```python
from build123d import *

# Parameters (mm, degrees)
F1_DEPTH  = 3.175
F2_R      = 3.556
F3_DEPTH  = 25.4
F4_DEPTH  = 25.4
F2_R_2    = 6.35
F5_DEPTH  = 25.4
F6_DEPTH  = 25.4
F7_DEPTH  = 25.4
F8_DEPTH  = 25.4
F9_R      = 18.9992
F9_R_2    = 1.8542
F10_DEPTH = 25.4


with BuildPart() as f1:
    # F0 (on Top) → F1 (new body)
    with BuildSketch(Plane.XY):
        Polygon((0, 31.75), (0, 101.6), (-444.5, 101.6), (-444.5, 31.75), (-412.75, 0), (-31.75, 0), align=None)
    extrude(amount=F1_DEPTH)

    # F2 (on face) → F3 (cut)
    with BuildSketch(Plane.XY.offset(3.175)):
        with Locations((-438.15, 50.8)):
            Circle(F2_R)
    extrude(amount=-F3_DEPTH, mode=Mode.SUBTRACT)

    # F2 (on face) → F4 (cut)
    with BuildSketch(Plane.XY.offset(3.175)):
        with Locations((-438.15, 76.2)):
            Circle(F2_R)
    extrude(amount=-F4_DEPTH, mode=Mode.SUBTRACT)

    # F2 (on face) → F5 (cut)
    with BuildSketch(Plane.XY.offset(3.175)):
        with Locations((-381, 31.75)):
            Circle(F2_R_2)
    extrude(amount=-F5_DEPTH, mode=Mode.SUBTRACT)

    # F2 (on face) → F6 (cut)
    with BuildSketch(Plane.XY.offset(3.175)):
        with Locations((-63.5, 31.75)):
            Circle(F2_R_2)
    extrude(amount=-F6_DEPTH, mode=Mode.SUBTRACT)

    # F2 (on face) → F7 (cut)
    with BuildSketch(Plane.XY.offset(3.175)):
        with Locations((-6.35, 76.2)):
            Circle(F2_R)
    extrude(amount=-F7_DEPTH, mode=Mode.SUBTRACT)

    # F2 (on face) → F8 (cut)
    with BuildSketch(Plane.XY.offset(3.175)):
        with Locations((-6.35, 50.8)):
            Circle(F2_R)
    extrude(amount=-F8_DEPTH, mode=Mode.SUBTRACT)

    # F9 (on face) → F10 (cut)
    with BuildSketch(Plane.XY.offset(3.175)):
        with Locations((-314.325, 31.75)):
            Circle(F9_R)
        with Locations((-338.328, 38.7604)):
            Circle(F9_R_2)
        with Locations((-290.322, 38.7604)):
            Circle(F9_R_2)
        with Locations((-130.175, 31.75)):
            Circle(F9_R)
        with Locations((-154.178, 38.7604)):
            Circle(F9_R_2)
        with Locations((-106.172, 38.7604)):
            Circle(F9_R_2)
    extrude(amount=-F10_DEPTH, mode=Mode.SUBTRACT)


solid = f1.part
```
Could you check a few things on this model? Use its own coordinates, in mm. Give positions to 0.01 mm unless a question says otherwise; leave off trailing zeros. Loops run counter-clockwise (first coordinate to the right, second up) from the corner with the lowest first, then second, coordinate; pieces in that order, holes last. Notation, with made-up numbers: (19.5, -16) -> (33.5, -16) arc R18 cw to (33.5, 15) -> close; hole circle Ø3 at (-31, 86.25). An arc over 180 degrees is marked (long way). Put each result on its own line as item: value.
(1) Imagine slicing it at A-A on x = -63.5. Write out the boundary of the cut face in (y, z) (3 decimals), plus the area to 3 significant figures.
Computed:
outline: (0, 0) -> (25.4, 0) -> (25.4, 3.175) -> (0, 3.175) -> close; (38.1, 0) -> (101.6, 0) -> (101.6, 3.175) -> (38.1, 3.175) -> close
area: 282 mm^2
(2) Please list where these lines run through material, in increasing order: probe 1 along X at (y, z) = (51.5, 3); probe 2 along Y at (x, z) = (-381, 2.3); probe 3 along Y at (x, z) = (-131, 1.3). Write a range as [from, to].
Computed:
probe 1: [-444.5, -441.64], [-434.66, -9.84], [-2.86, 0]
probe 2: [0, 25.4], [38.1, 101.6]
probe 3: [0, 12.77], [50.73, 101.6]
(3) Imagine slicing it at B-B on z = 1.45. State how many separate pieces and enclosed holes the cut face has, plus the area to 3 significant figures.
Computed:
separate pieces: 1
enclosed holes: 12
area: 41,400 mm^2
(4) Thinking about a two-plate mould opening in Y: for faces 1 (the face through (-225, 52, 0)), 2 (the face through (-112.625, 24.473, 1.61)), 3 (the face through (-428.85, 16.1, 1.57)), which applies, pulls with the +Y half, pulls with the -Y half, needs draft (parallel to the pull), parting line crosses it, or undercut?
Computed:
face 1: needs draft
face 2: undercut
face 3: pulls with the -Y half
